```python
from build123d import *

# Parameters (mm, degrees)
EXTRUDE_1_DEPTH = 4
SKETCH_2_R      = 2.1
EXTRUDE_2_DEPTH = 18.44


with BuildPart() as part:
    # Эскиз1 → Бобышка-Вытянуть1 (new body)
    with BuildSketch(Plane(origin=(0, 0, 0), x_dir=(1, 0, 0), z_dir=(0, 1, 0))):
        with BuildLine():
            Line((-1.004775086, -8.439280951), (-0.521670756, -8.568728366))
            ThreePointArc((-0.521670756, -8.568728366), (0.439799359, -8.436274341), (1.016677121, -7.655773926))
            ThreePointArc((1.016677121, -7.655773926), (1.93125128, 0), (1.016677121, 7.655773926))
            ThreePointArc((1.016677121, 7.655773926), (0.439799359, 8.436274341), (-0.521670756, 8.568728366))
            Line((-0.521670756, 8.568728366), (-1.004775086, 8.439280951))
            ThreePointArc((-1.004775086, 8.439280951), (-1.756080004, 7.870029772), (-1.8961902, 6.937895063))
            ThreePointArc((-1.8961902, 6.937895063), (-1.06874872, 0), (-1.8961902, -6.937895063))
            ThreePointArc((-1.8961902, -6.937895063), (-1.756080004, -7.870029772), (-1.004775086, -8.439280951))
        make_face()
    extrude(amount=EXTRUDE_1_DEPTH)

    # Эскиз2 → Бобышка-Вытянуть2 (add)
    with BuildSketch(Plane(origin=(0, 2, 0), x_dir=(1, 0, 0), z_dir=(0, 1, 0))):
        with Locations(Location((0.43125128, 0, 0), (0, 0, 45.757566992))):
            Circle(SKETCH_2_R)
    extrude(amount=EXTRUDE_2_DEPTH)


solid = part.part
```
Geometry check sheet. Reference: the model listing, model coordinates, mm. A direction names the side the tool comes from. Coordinates: 2 decimals unless noted, no trailing zeros. Order: outer loops, then holes, each group sorted by start corner. A loop starts at its lowest first (then second) coordinate and runs counter-clockwise, first axis right, second up. Notation, with made-up numbers: (23, -21) - (59, -21) arc R19 ccw to (59, 2) - close; hole circle Ø11 at (7, -33.75). An arc over 180 degrees is marked (long way). Use one line per item in the form item = value.
1. Section check A-A (z = 0). Record the boundary of the cut face in (x, y), then the cut area to 3 significant figures.
Here are the results:
outline = (-1.67, 2) - (-1.07, 2) - (-1.07, 0) - (1.93, 0) - (1.93, 2) - (2.53, 2) - (2.53, 20.44) - (-1.67, 20.44) - close
area = 83.4 mm²
2. Scan lines: line 1 (Y direction, x = 0.75, z = -3.75); line 2 (Z direction, x = 1.9, y = 17.75); line 3 (Y direction, x = 2.05, z = -0.25). Record each from-to range of solid material in increasing order.
Here are the results:
line_1 = 0 to 4
line_2 = -1.5 to 1.5
line_3 = 2 to 20.44
3. Section check C-C (x = 0.4). Record the boundary of the cut face in (y, z), then the cut area to 3 significant figures.
Here are the results:
outline = (0, -8.46) - (4, -8.46) - (4, -2.1) - (20.44, -2.1) - (20.44, 2.1) - (4, 2.1) - (4, 8.46) - (0, 8.46) - close
area = 137 mm²
4. Gauge pin test, flat ends, axial feed: pin 1 (0.7 mm diameter, centred on x = -1.5, z = 0, fed in from -Y); pin 2 (1.9 mm diameter, centred on x = 0, z = -3.5, fed in from +Y); pin 3 (1.5 mm diameter, centred on x = 1, y = 3.5, fed in from -Z). Record the tip position at first contact, or that the pin passes through.
Here are the results:
pin_1 = 2
pin_2 = 4
pin_3 = -8.53
5. Section check B-B (y = 12). Record the boundary of the cut face in (x, z).
Here are the results:
outline = circle Ø4.2 at (0.43, 0)
6. Section check D-D (z = 6). Record the boundary of the cut face in (x, y).
Here are the results:
outline = (-1.69, 0) - (1.37, 0) - (1.37, 4) - (-1.69, 4) - close
7. Access from +Z, -Z, +X, -X, +Y, -Y to the whole of each face (thin tool, end or side, straight path). Record for faces 1 (the face through (1.377, 11.091, -1.875)), 2 (the face through (0, 20.44, 0)).
Here are the results:
face_1 = +Y
face_2 = +Z, -Z, +X, -X, +Y
